Study the drawing (mm; zero at the part's minimum x, y, z) and answer. Coordinates: 2 decimals unless noted, no trailing zeros. Order: outer loops, then holes, each group sorted by start corner. A loop starts at its lowest first (then second) coordinate and runs counter-clockwise, first axis right, second up.
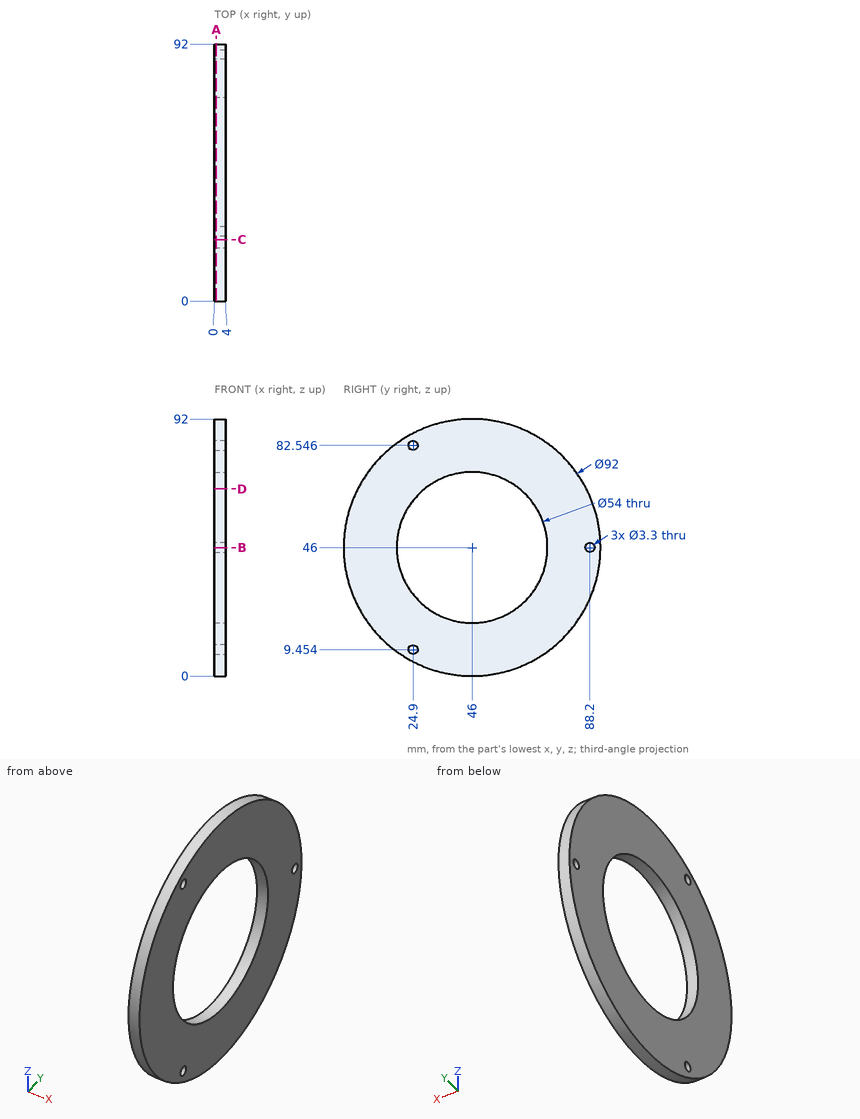
(1) Given pin 1 Ø3 at (y, z) = (24.9, 82.55) entering from +X; pin 2 Ø1 at (x, y) = (1, 9.5) entering from -Z (1 decimal); pin 3 Ø1.5 at (x, z) = (2, 20) entering from -Y, each flat-ended and moving along its own axis, determine where each tip first touches the part or whether it passes through.
(2) Find the intervals of material crossed by probe 1 along Y at (x, z) = (3.15, 46); probe 2 along Z at (x, y) = (1.1, 24.9) (1 decimal); probe 3 along Y at (x, z) = (3.7, 47.5) (1 decimal), in increasing order.
(3) Find section A-A on x = 0.7. Determine the outline of the cut face in (y, z).
(4) Find section B-B on z = 46. Determine the outline of the cut face in (x, y).
(5) Find section C-C on y = 22. Determine the outline of the cut face in (x, z), then the cut area to 3 significant figures.
(6) Find section D-D on z = 67. Determine the outline of the cut face in (x, y).
Resolved:
1. pin 1: passes through
1. pin 2: stops at z = 17.4
1. pin 3: stops at y = 7.55
2. probe 1: y = 0 to 19, 73 to 86.55, 89.85 to 92
2. probe 2: z = 5.1 to 7.8, 11.1 to 29.2, 62.8 to 80.9, 84.2 to 86.9
2. probe 3: y = 0 to 19, 73 to 87.5, 88.9 to 92
3. outline: circle Ø92 at (46, 46); hole circle Ø54 at (46, 46); hole circle Ø3.3 at (24.9, 9.45); hole circle Ø3.3 at (24.9, 82.55); hole circle Ø3.3 at (88.2, 46)
4. outline: (0, 0) - (4, 0) - (4, 19) - (0, 19) - close; (0, 73) - (4, 73) - (4, 86.55) - (0, 86.55) - close; (0, 89.85) - (4, 89.85) - (4, 92) - (0, 92) - close
5. outline: (0, 6.76) - (4, 6.76) - (4, 33.63) - (0, 33.63) - close; (0, 58.37) - (4, 58.37) - (4, 85.24) - (0, 85.24) - close
5. area: 215 mm2
6. outline: (0, 5.07) - (4, 5.07) - (4, 29.03) - (0, 29.03) - close; (0, 62.97) - (4, 62.97) - (4, 86.93) - (0, 86.93) - close
